from build123d import *

# Parameters (mm, degrees)
SKETCH1_W           = 22.86
SKETCH1_H           = 15.24
BOSS_EXTRUDE1_DEPTH = 5.08
SKETCH3_W           = 2.413
SKETCH3_H           = 15.24
BOSS_EXTRUDE3_DEPTH = 5.207
SKETCH4_W           = 22.86
SKETCH4_H           = 15.24
SKETCH4_R           = 2.54
BOSS_EXTRUDE4_DEPTH = 2.54
SKETCH5_W           = 22.86
SKETCH5_H           = 15.24
SKETCH5_R           = 2.54
BOSS_EXTRUDE5_DEPTH = 1.27
FILLET1_R           = 5.08


with BuildPart() as part:
    # Sketch1 → Boss-Extrude1 (new body)
    with BuildSketch(Plane(origin=(0, 0, 0), x_dir=(1, 0, 0), z_dir=(0, 1, 0))):
        Rectangle(SKETCH1_W, SKETCH1_H)
        Polygon((5.572584798, 0), (2.786292399, 4.826), (-2.786292399, 4.826), (-5.572584798, 0), (-2.786292399, -4.826), (2.786292399, -4.826), align=None, mode=Mode.SUBTRACT)
    extrude(amount=BOSS_EXTRUDE1_DEPTH)

    # Sketch3 → Boss-Extrude3 (add)
    with BuildSketch(Plane(origin=(0, 5.08, 0), x_dir=(1, 0, 0), z_dir=(0, 1, 0))):
        with Locations((-10.2235, 0)):
            Rectangle(SKETCH3_W, SKETCH3_H)
        with Locations((10.2235, 0)):
            Rectangle(SKETCH3_W, SKETCH3_H)
    extrude(amount=BOSS_EXTRUDE3_DEPTH)

    # Sketch4 → Boss-Extrude4 (add)
    with BuildSketch(Plane(origin=(0, 10.287, 0), x_dir=(1, 0, 0), z_dir=(0, 1, 0))):
        Rectangle(SKETCH4_W, SKETCH4_H)
        Circle(SKETCH4_R, mode=Mode.SUBTRACT)
    extrude(amount=BOSS_EXTRUDE4_DEPTH)

    # Sketch5 → Boss-Extrude5 (add)
    with BuildSketch(Plane.XZ):
        Rectangle(SKETCH5_W, SKETCH5_H)
        Circle(SKETCH5_R, mode=Mode.SUBTRACT)
    extrude(amount=BOSS_EXTRUDE5_DEPTH)

    # Fillet1
    fillet1_edges = [part.edges().sort_by_distance(p)[0] for p in [
        (-11.43, 12.827, 0),
        (11.43, 12.827, 0),
        (-11.43, -1.27, 0),
        (11.43, -1.27, 0),
    ]]
    fillet(fillet1_edges, radius=FILLET1_R)


solid = part.part
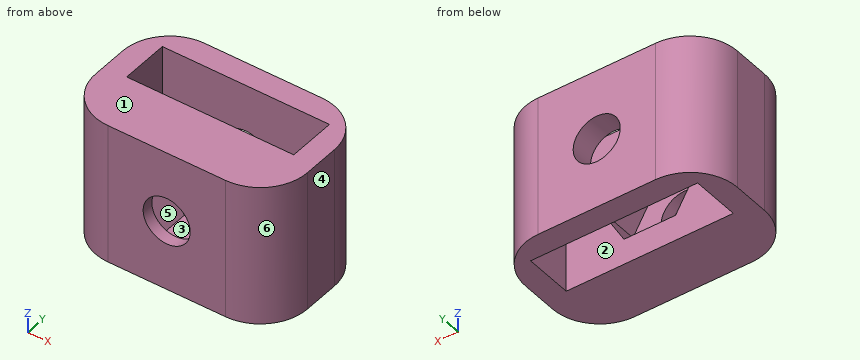
Check sheet for the modelled part. Datum: model origin and axes. Units: mm. Face numbers are marked on the shaded views. A direction names the side the tool comes from. Give positions to 0.01 mm unless a question says otherwise; leave off trailing zeros. Write each loop counter-clockwise with the first axis right and the second up, starting at its lowest first coordinate (ties: lowest second). Pieces come first, ordered by that corner, then holes. Notation, with made-up numbers: M 33.5,31.25 L 64.5,31.25 A10 cw 64.5,50.25 Z; hole C 27.5,77 d2. An arc over 180 degrees is marked long. Use one line per item in the form item = value.
(1) Tool access check on the marked faces 1, 2 and 3. Record the directions out of +Z, -Z, +X, -X, +Y, -Y that give a thin tool (end or side, any length) a straight path to the whole face; none if there is none.
Answer block:
face_1 = +Z, +X, -X, +Y, -Y
face_2 = +Z, -Z
face_3 = none
(2) Depth check by flat-ended pin: P1, Ø1.5, axis at y = 2, z = -3.5, coming from the +X side; P2, Ø1, axis at y = 9, z = 5, coming from the -X side. Enter the tip coordinate at first touch or a pass-through.
Answer block:
P1 = 11.32
P2 = -11.37
(3) Draft check along Y on the marked faces 4, 5 and 6. Enter one of: pulls with the +Y half, pulls with the -Y half, needs draft (parallel to the pull), parting line crosses it, or undercut.
Answer block:
face_4 = needs draft
face_5 = undercut
face_6 = pulls with the -Y half
(4) Section check A-A on y = 7. Record the boundary of the cut face in (x, z).
Answer block:
outline = M -11.43,-7.62 L -9.02,-7.62 L -9.02,7.62 L -11.43,7.62 Z; M 9.02,-7.62 L 11.43,-7.62 L 11.43,7.62 L 9.02,7.62 Z
(5) Material ranges on line 1 along Y through (x, z) = (-1.75, -4.75); line 2 along Y through (x, z) = (6.25, 1.75); line 3 along Z through (x, y) = (0, -0.65), recorded low to high.
Answer block:
line_1 = -1.27 to 0, 10.29 to 12.83
line_2 = -1.27 to 5.08, 10.29 to 12.83
line_3 = -7.62 to -2.54, 2.54 to 7.62
(6) Section check C-C on z = 6.25. Record the boundary of the cut face in (x, y).
Answer block:
outline = M -11.43,3.81 A5.08 ccw -6.35,-1.27 L 6.35,-1.27 A5.08 ccw 11.43,3.81 L 11.43,7.75 A5.08 ccw 6.35,12.83 L -6.35,12.83 A5.08 ccw -11.43,7.75 Z; hole M -9.02,5.08 L 9.02,5.08 L 9.02,10.29 L -9.02,10.29 Z
(7) Section check D-D on x = 7.5. Record the boundary of the cut face in (y, z).
Answer block:
outline = M -1.14,-7.62 L 5.08,-7.62 L 5.08,7.62 L -1.14,7.62 Z; M 10.29,-7.62 L 12.7,-7.62 L 12.7,7.62 L 10.29,7.62 Z
(8) Section check B-B on x = 0. Record the boundary of the cut face in (y, z).
Answer block:
outline = M -1.27,-7.62 L 5.08,-7.62 L 5.08,-4.83 L 0,-4.83 L 0,-2.54 L -1.27,-2.54 Z; M -1.27,2.54 L 0,2.54 L 0,4.83 L 5.08,4.83 L 5.08,7.62 L -1.27,7.62 Z; M 10.29,-7.62 L 12.83,-7.62 L 12.83,-2.54 L 10.29,-2.54 Z; M 10.29,2.54 L 12.83,2.54 L 12.83,7.62 L 10.29,7.62 Z
